The listing builds one solid part. Answer for the finished solid, in the listing's coordinates (mm). A direction names the side the tool comes from. Give positions to 0.01 mm unless a question says otherwise; leave off trailing zeros. Order: outer loops, then holes, each group sorted by start corner. A loop starts at its lowest first (then second) coordinate and runs counter-clockwise, first axis right, second up.
Autodesk Inventor part; units mm, degrees
ref_plane "YZ Plane" through (0, 0, 0) normal (1, 0, 0) x (0, 1, 0)
ref_plane "XZ Plane" through (0, 0, 0) normal (0, 1, 0) x (-1, 0, 0)
ref_plane "XY Plane" through (0, 0, 0) normal (0, 0, 1) x (1, 0, 0)
sketch "Sketch1" plane through (0, 0, 0) normal (0, 0, 1) x (1, 0, 0)
  line L0 (-2.5, 9) -> (2.5, 9)
  line L1 (2.5, 9) -> (2.5, -9)
  line L2 (2.5, -9) -> (-2.5, -9)
  line L3 (-2.5, -9) -> (-2.5, 9)
  line L4 (-2.5, 9) -> (2.5, -9) construction
  line L5 (2.5, 9) -> (-2.5, -9) construction
  line L6 (-15, 0) -> (-7.5, 0)
  line L7 (-7.5, 0) -> (-7.5, -3)
  line L8 (-7.5, -3) -> (-15, -3)
  line L9 (-15, -3) -> (-15, 0)
  line L10 (7.5, 0) -> (15, 0)
  line L11 (15, 0) -> (15, -3)
  line L12 (15, -3) -> (7.5, -3)
  line L13 (7.5, -3) -> (7.5, 0)
  line L14 (7.5, -3) -> (7.5, -6)
  line L15 (7.5, -6) -> (15, -6)
  line L16 (15, -6) -> (15, -3)
  line L17 (-7.5, -3) -> (-7.5, -6)
  line L18 (-7.5, -6) -> (-15, -6)
  line L19 (-15, -6) -> (-15, -3)
  line L20 (-7.5, -1.5) -> (7.5, -1.5) construction
  line L21 (-1, -9) -> (-2.5, -4.878784)
  line L22 (1, -9) -> (2.5, -4.878784)
  arc A0 (-2.5, -4.678784) -> (-7.5, -5.8) centre (-4.32787, -8.236717) ccw construction
  arc A1 (-2.408606, -4.500887) -> (-7.658606, -5.678164) centre (-4.32787, -8.236717) ccw
  arc A2 (-2.591394, -4.856681) -> (-7.341394, -5.921836) centre (-4.32787, -8.236717) ccw
  arc A3 (-2.591394, -4.856681) -> (-2.408606, -4.500887) centre (-2.5, -4.678784) ccw
  arc A4 (-7.658606, -5.678164) -> (-7.341394, -5.921836) centre (-7.5, -5.8) ccw
  arc A5 (7.5, -5.8) -> (2.5, -4.678784) centre (4.32787, -8.236717) ccw construction
  arc A6 (7.658606, -5.678164) -> (2.408606, -4.500887) centre (4.32787, -8.236717) ccw
  arc A7 (7.341394, -5.921836) -> (2.591394, -4.856681) centre (4.32787, -8.236717) ccw
  arc A8 (7.341394, -5.921836) -> (7.658606, -5.678164) centre (7.5, -5.8) ccw
  arc A9 (2.408606, -4.500887) -> (2.591394, -4.856681) centre (2.5, -4.678784) ccw
  arc A10 (-2.5, -1.678784) -> (-7.5, -2.8) centre (-4.32787, -5.236717) ccw construction
  arc A11 (-2.408606, -1.500887) -> (-7.658606, -2.678164) centre (-4.32787, -5.236717) ccw
  arc A12 (-2.591394, -1.856681) -> (-7.341394, -2.921836) centre (-4.32787, -5.236717) ccw
  arc A13 (-2.591394, -1.856681) -> (-2.408606, -1.500887) centre (-2.5, -1.678784) ccw
  arc A14 (-7.658606, -2.678164) -> (-7.341394, -2.921836) centre (-7.5, -2.8) ccw
  arc A15 (7.5, -2.8) -> (2.5, -1.678784) centre (4.32787, -5.236717) ccw construction
  arc A16 (7.658606, -2.678164) -> (2.408606, -1.500887) centre (4.32787, -5.236717) ccw
  arc A17 (7.341394, -2.921836) -> (2.591394, -1.856681) centre (4.32787, -5.236717) ccw
  arc A18 (7.341394, -2.921836) -> (7.658606, -2.678164) centre (7.5, -2.8) ccw
  arc A19 (2.408606, -1.500887) -> (2.591394, -1.856681) centre (2.5, -1.678784) ccw
  point P0 (0, 0)
  point P1 (0, -1.5)
  point P2 (-7.5, -5.483975)
  point P3 (-2.5, -1.878784)
  point P4 (-2.5, -4.45533)
  point P5 (7.5, -5.483975)
  point P6 (2.5, -4.45533)
  point P7 (2.5, -1.878784)
  point P8 (7.5, -2.483975)
  point P9 (2.5, -1.45533)
  point P10 (-2.5, -1.45533)
  point P11 (-7.5, -2.483975)
  dimension "d0" = 5
  dimension "d1" = 18
  dimension "d2" = 30
  dimension "d3" = 3
  dimension "d4" = 3
  dimension "d5" = 5
  dimension "d8" = 9
  dimension "d9" = 3
  dimension "d10" = 2
  dimension "d11" = 20
  dimension "d12" = 0.4
  dimension "d13" = 4
  dimension "d14" = 3
sketch "Sketch1 outline for Extrusion1" plane through (0, 0, 0) normal (0, 0, 1) x (1, 0, 0)
  arc A0 (-7.5, -6) -> (-7.341394, -5.921836) centre (-7.5, -5.8) ccw
  line L0 (-15, -6) -> (-7.5, -6)
  arc A1 (-7.341394, -5.921836) -> (-2.591394, -4.856681) centre (-4.32787, -8.236717) cw
  line L1 (-15, -3) -> (-15, -6)
  arc A2 (-2.591394, -4.856681) -> (-2.5, -4.878784) centre (-2.5, -4.678784) ccw
  line L2 (-15, 0) -> (-15, -3)
  line L3 (-2.5, -4.878784) -> (-1, -9)
  line L4 (-7.5, 0) -> (-15, 0)
  line L5 (-1, -9) -> (1, -9)
  line L6 (-7.5, -2.483975) -> (-7.5, 0)
  line L7 (1, -9) -> (2.5, -4.878784)
  arc A3 (-2.5, -1.45533) -> (-7.5, -2.483975) centre (-4.32787, -5.236717) ccw
  arc A4 (2.5, -4.878784) -> (2.591394, -4.856681) centre (2.5, -4.678784) ccw
  line L8 (-2.5, 9) -> (-2.5, -1.45533)
  arc A5 (2.591394, -4.856681) -> (7.341394, -5.921836) centre (4.32787, -8.236717) cw
  line L9 (2.5, 9) -> (-2.5, 9)
  arc A6 (7.341394, -5.921836) -> (7.5, -6) centre (7.5, -5.8) ccw
  line L10 (2.5, -1.45533) -> (2.5, 9)
  line L11 (7.5, -6) -> (15, -6)
  arc A7 (7.5, -2.483975) -> (2.5, -1.45533) centre (4.32787, -5.236717) ccw
  line L12 (15, -6) -> (15, -3)
  line L13 (7.5, 0) -> (7.5, -2.483975)
  line L14 (15, -3) -> (15, 0)
  line L15 (15, 0) -> (7.5, 0)
  line L16 (-7.5, -5.483975) -> (-7.5, -3)
  arc A8 (-2.5, -4.45533) -> (-7.5, -5.483975) centre (-4.32787, -8.236717) ccw
  line L17 (-2.5, -1.878784) -> (-2.5, -4.45533)
  arc A9 (-2.591394, -1.856681) -> (-2.5, -1.878784) centre (-2.5, -1.678784) ccw
  arc A10 (-7.341394, -2.921836) -> (-2.591394, -1.856681) centre (-4.32787, -5.236717) cw
  arc A11 (-7.5, -3) -> (-7.341394, -2.921836) centre (-7.5, -2.8) ccw
  arc A12 (7.5, -5.483975) -> (2.5, -4.45533) centre (4.32787, -8.236717) ccw
  line L18 (7.5, -3) -> (7.5, -5.483975)
  arc A13 (7.341394, -2.921836) -> (7.5, -3) centre (7.5, -2.8) ccw
  arc A14 (2.591394, -1.856681) -> (7.341394, -2.921836) centre (4.32787, -5.236717) cw
  arc A15 (2.5, -1.878784) -> (2.591394, -1.856681) centre (2.5, -1.678784) ccw
  line L19 (2.5, -4.45533) -> (2.5, -1.878784)
extrude "Extrusion1" add sketch "Sketch1 outline for Extrusion1" along normal blind 8
chamfer "Chamfer1" distance 3 angle 45 1 edges at (0, -9, 0) measured on face at (-0.3333, -9, 2.6667)
chamfer "Chamfer2" distance 3 angle 45 1 edges at (0, -9, 8) measured on face at (-0.3333, -9, 4.6667)
fillet "Fillet1" radius 0.2 14 edges at (-7.5, -2.484, 4) (-7.5, -3, 4) (-7.5, -5.484, 4) (-2.5, -4.8788, 4) (-2.5, -4.4553, 4) (-2.5, -1.8788, 4) (-2.5, -1.4553, 4) (2.5, -1.4553, 4) (2.5, -1.8788, 4) (2.5, -4.4553, 4) (2.5, -4.8788, 4) (7.5, -5.484, 4) (7.5, -3, 4) (7.5, -2.484, 4)
fillet "Fillet2" radius 0.4 12 edges at (-15, 0, 4) (-15, -3, 4) (15, -3, 4) (15, 0, 4) (7.5, 0, 4) (15, -6, 4) (-15, -6, 4) (-7.5, 0, 4) (-2.5, 9, 4) (2.5, 9, 4) (-1, -9, 4) (1, -9, 4)
sketch "Sketch3" plane through (-14.6, 0, 0) normal (0, 1, 0) x (1, 0, 0)
  line L0 (3.35, -4) -> (25.85, -4) construction
  line L1 (16.7, 0) -> (12.5, 0)
  line L2 (29.2, 0) -> (29.2, -8)
  line L3 (6.7, -8) -> (0, -8)
  point P0 (14.6, 0)
  point P1 (14.6, -4)
  point P2 (14.6, 0)
  point P3 (29.2, -4)
  point P4 (3.35, -8)
hole "Hole2" at (-11.25, 0, 4) at (11.25, 0, 4) direction (0, -1, 0) diameter 4 end through all
sketch "Sketch4" plane through (-2.1, 9, 0) normal (0, 1, 0) x (1, 0, 0)
  line L0 (-12.9, 0) -> (-0.4, 0)
  line L1 (-0.4, 0) -> (-0.4, -8)
  line L2 (-0.4, -8) -> (-12.9, -8)
  line L3 (-12.9, -8) -> (-12.9, 0)
  line L4 (-5.8, -8) -> (-12.5, -8)
  line L5 (-5.8, 0) -> (-12.5, 0)
  line L6 (-12.9, 0) -> (-12.9, -8)
  line L7 (-0.4, 0) -> (-0.4, -8)
  point P0 (2.1, 0)
sketch "Sketch4 outline for Extrusion2" plane through (-2.1, 9, 0) normal (0, 1, 0) x (1, 0, 0)
  line L0 (-12.9, 0) -> (-12.9, -8)
  line L1 (-0.4, 0) -> (-12.9, 0)
  line L2 (-0.4, -8) -> (-0.4, 0)
  line L3 (-12.9, -8) -> (-0.4, -8)
extrude "Extrusion2" cut sketch "Sketch4 outline for Extrusion2" against normal through all
equation "\"d4\" = d3"
properties part number "Actuator 2"
1) For a pull along Y with two mould halves and no side action, classify faces 6 (the flat face through (9, -6, 5)), 7 (the flat face through (2.5, 4, 4)), 8 (the flat face through (7.5, -4, 4)) as +Y half, -Y half, draft (parallel to the pull), parting line (faces both ways), or undercut.
Geometry says:
face 6: -Y half
face 7: draft
face 8: undercut
2) Find section A-A (x = 11.25). Write down the section's boundary in (y, z).
Geometry says:
outline: (-6, 0) - (0, 0) - (0, 2) - (-6, 2) - close; (-6, 6) - (0, 6) - (0, 8) - (-6, 8) - close
3) Find section B-B (y = 7). Write down the section's boundary in (x, z), then the cut area to 3 significant figures.
Geometry says:
outline: (-2.5, 0) - (2.5, 0) - (2.5, 8) - (-2.5, 8) - close
area: 40.0 mm2
4) Find section D-D (x = 5.75). Write down the section's boundary in (y, z), then the cut area to 3 significant figures.
Geometry says:
outline: (-4.71, 0) - (-4.28, 0) - (-4.28, 8) - (-4.71, 8) - close; (-1.71, 0) - (-1.28, 0) - (-1.28, 8) - (-1.71, 8) - close
area: 6.85 mm2
5) Find section C-C (z = 4.75). Count the separate pieces of the cut face and the enclosed holes in it, then the cut area to 3 significant figures.
Geometry says:
separate pieces: 2
enclosed holes: 1
area: 111 mm2
6) Given P1, Ø3, axis at y = -7, z = 3, coming from the -X side; P2, Ø10, axis at x = 8.5, y = -6.5, coming from the +Z side; P3, Ø2.5, axis at y = 2.5, z = 3, coming from the +X side; P4, Ø2, axis at x = 11.5, z = 3, coming from the +Y side, each flat-ended and moving along its own axis, determine where each tip first touches the part or whether it passes through.
Geometry says:
P1: stops at x = -2.27
P2: stops at z = 8
P3: stops at x = 2.5
P4: stops at y = 0
7) Straight lines are drawn through the part: probe 1 along Z at (x, y) = (11.25, -3.75); probe 2 along X at (y, z) = (-1.4, 4); probe 3 along X at (y, z) = (-4.75, 5.25). For each, find the intervals that lie inside material, in ascending order.
Geometry says:
probe 1: z = 0 to 2, 6 to 8
probe 2: x = -2.5 to 6.04, 7.5 to 9.25, 13.25 to 15
probe 3: x = -2.5 to 2.82, 5.84 to 6.67, 7.5 to 9.69, 12.81 to 15
8) A tool of negligible diameter and unlimited length cuts with its end or side. For faces 1 (the cylindrical face through (5.05, -4.1, 3.94)), 2 (the flat face through (1.92, -6.47, 3.94)), 3 (the flat face through (0, 9, 4)), 4 (the flat face through (-1.94, -6.42, 3.94)), 5 (the flat face through (7.5, -1, 4)), from which of +Z, -Z, +X, -X, +Y, -Y can it reach the whole face along a straight path? Write none if from no direction.
Geometry says:
face 1: +Z, -Z
face 2: +Z, -Z, -Y
face 3: +Z, -Z, +X, -X, +Y
face 4: +Z, -Z, -X, -Y
face 5: +Z, -Z, +Y
